Read the model definition and answer for the solid it produces. Units are mm, in the model's axes. Face numbers are marked on the shaded views. A direction names the side the tool comes from. Round coordinates to 2 decimals unless told otherwise and drop trailing zeros. Order: outer loops, then holes, each group sorted by start corner. A loop starts at its lowest first (then second) coordinate and runs counter-clockwise, first axis right, second up. Notation, with made-up numbers: (40, 88.5) -> (68, 88.5) arc R29 cw to (68, 119.5) -> close; hole circle Ø7 at (36, -7). An arc over 180 degrees is marked (long way). Answer as a JSON object with one key per item and string values. Group by question number.
Item 1: Section D-D, the plane y = 48 is taken. Write down the section's boundary in (x, z), plus the area to 3 significant figures.
Item 2: Section C-C, the plane y = 17 is taken. Write down the section's boundary in (x, z).
Item 3: Consider probe 1 along Y at (x, z) = (0, 78); probe 2 along Y at (x, z) = (1.5, 75); probe 3 along Z at (x, y) = (39.5, 23). Determine where each line is inside the solid, lowest interval first. Write a range as from..to.
Item 4: For the marked faces 4 and 5, determine the directions among +Z, -Z, +X, -X, +Y, -Y from which every point of the face is accessible in a straight line to the end or side of a thin tool.
Item 5: The mould has two halves that part along Y. Classify the marked faces 1, 2 and 3: pulls with the +Y half, pulls with the -Y half, needs draft (parallel to the pull), parting line crosses it, or undercut.
Item 6: Given P1, Ø7, axis at x = -48, y = 0, coming from the +Z side; P2, Ø8, axis at x = -36.5, z = 46, coming from the -Y side; P3, Ø12, axis at y = -8.5, z = 16.5, coming from the -X side; P4, Ø6, axis at y = 31.5, z = 48, coming from the +X side, each flat-ended and moving along its own axis, determine where each tip first touches the part or whether it passes through.
Item 7: Section A-A, the plane y = 0 is taken. Count the separate pieces of the cut face and the enclosed holes in it, plus the area to 3 significant figures.
Item 8: Section B-B, the plane x = -12 is taken. Write down the section's boundary in (y, z).
from build123d import *

# Parameters (mm, degrees)
SKETCH1_R               = 38
SKETCH1_R_2             = 36.8
BOSS_EXTRUDE1_DEPTH     = 80
CUT_EXTRUDE1_DEPTH      = 97.374270425
CUT_EXTRUDE1_DEPTH_BACK = 97.374270425
SKETCH2_R               = 3.5
BOSS_EXTRUDE2_START     = -3
SKETCH3_R               = 58
SKETCH3_R_2             = 38
SKETCH3_R_3             = 4.5
BOSS_EXTRUDE2_DEPTH     = 3
SKETCH4_R               = 58
SKETCH4_R_2             = 38
SKETCH4_R_3             = 4.5
BOSS_EXTRUDE3_DEPTH     = 3


with BuildPart() as part:
    # Sketch1 → Boss-Extrude1 (new body)
    with BuildSketch(Plane.XY):
        Circle(SKETCH1_R)
        Circle(SKETCH1_R_2, mode=Mode.SUBTRACT)
    extrude(amount=BOSS_EXTRUDE1_DEPTH)

    # Sketch2 → Cut-Extrude1 (cut, two sides: drawn at the far end of the back side and taken through both)
    with BuildSketch(Plane(origin=(0, 0, 0), x_dir=(1, 0, 0), z_dir=(0, 1, 0)).offset(-CUT_EXTRUDE1_DEPTH_BACK)):
        with Locations(Location((0, -40, 0), (0, 0, 270))):
            Circle(SKETCH2_R)
    extrude(amount=CUT_EXTRUDE1_DEPTH + CUT_EXTRUDE1_DEPTH_BACK, mode=Mode.SUBTRACT)

    # Sketch3 → Boss-Extrude2 (add)
    with BuildSketch(Plane.XY.offset(80).offset(BOSS_EXTRUDE2_START)):
        Circle(SKETCH3_R)
        Circle(SKETCH3_R_2, mode=Mode.SUBTRACT)
        with Locations((-48, 0)):
            Circle(SKETCH3_R_3, mode=Mode.SUBTRACT)
        with Locations((0, 48)):
            Circle(SKETCH3_R_3, mode=Mode.SUBTRACT)
        with Locations((48, 0)):
            Circle(SKETCH3_R_3, mode=Mode.SUBTRACT)
        with Locations((0, -48)):
            Circle(SKETCH3_R_3, mode=Mode.SUBTRACT)
    extrude(amount=BOSS_EXTRUDE2_DEPTH)

    # Sketch4 → Boss-Extrude3 (add)
    with BuildSketch(Plane(origin=(0, 0, 0), x_dir=(-1, 0, 0), z_dir=(0, 0, -1))):
        with Locations(Location((0, 0, 0), (0, 0, 180))):
            Circle(SKETCH4_R)
        Circle(SKETCH4_R_2, mode=Mode.SUBTRACT)
        with Locations(Location((48, 0, 0), (0, 0, 180))):
            Circle(SKETCH4_R_3, mode=Mode.SUBTRACT)
        with Locations(Location((0, -48, 0), (0, 0, 180))):
            Circle(SKETCH4_R_3, mode=Mode.SUBTRACT)
        with Locations(Location((-48, 0, 0), (0, 0, 180))):
            Circle(SKETCH4_R_3, mode=Mode.SUBTRACT)
        with Locations(Location((0, 48, 0), (0, 0, 180))):
            Circle(SKETCH4_R_3, mode=Mode.SUBTRACT)
    extrude(amount=-BOSS_EXTRUDE3_DEPTH)


solid = part.part
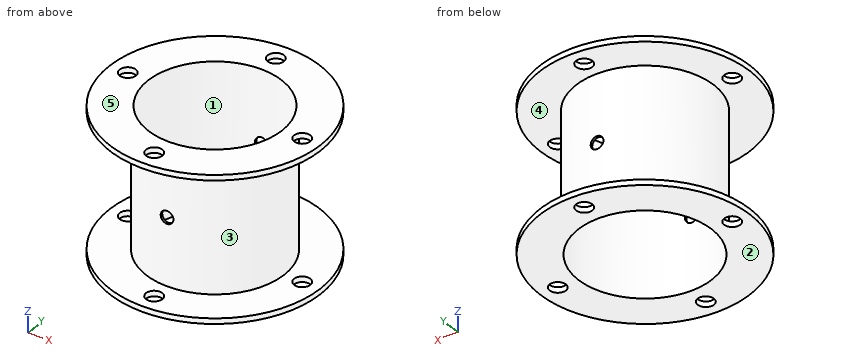
Values found:
{
 "1": {"outline": "(-32.56, 0) -> (-4.5, 0) -> (-4.5, 3) -> (-32.56, 3) -> close; (-32.56, 77) -> (-4.5, 77) -> (-4.5, 80) -> (-32.56, 80) -> close; (4.5, 0) -> (32.56, 0) -> (32.56, 3) -> (4.5, 3) -> close; (4.5, 77) -> (32.56, 77) -> (32.56, 80) -> (4.5, 80) -> close", "area": "337 mm2"},
 "2": {"outline": "(-55.45, 0) -> (-32.64, 0) -> (-32.64, 80) -> (-55.45, 80) -> (-55.45, 77) -> (-33.99, 77) -> (-33.99, 3) -> (-55.45, 3) -> close; (32.64, 0) -> (55.45, 0) -> (55.45, 3) -> (33.99, 3) -> (33.99, 77) -> (55.45, 77) -> (55.45, 80) -> (32.64, 80) -> close"},
 "3": {"probe 1": "-58..-52.5, -43.5..-36.8, 36.8..43.5, 52.5..58", "probe 2": "-37.97..-36.77, 36.77..37.97", "probe 3": "0..3, 77..80"},
 "4": {"face 4": "none", "face 5": "+Z, +X, -X, +Y, -Y"},
 "5": {"face 1": "undercut", "face 2": "needs draft", "face 3": "parting line crosses it"},
 "6": {"P1": "through", "P2": "y = -19.69", "P3": "x = -37.92", "P4": "x = 25.13"},
 "7": {"separate pieces": "6", "enclosed holes": "0", "area": "324 mm2"},
 "8": {"outline": "(-56.75, 0) -> (-34.79, 0) -> (-34.79, 80) -> (-56.75, 80) -> (-56.75, 77) -> (-36.06, 77) -> (-36.06, 3) -> (-56.75, 3) -> close; (34.79, 0) -> (56.75, 0) -> (56.75, 3) -> (36.06, 3) -> (36.06, 77) -> (56.75, 77) -> (56.75, 80) -> (34.79, 80) -> close"}
}
